Geometry check sheet. Reference: the model listing, model coordinates, mm. Coordinates: 2 decimals unless noted, no trailing zeros. Write each loop counter-clockwise with the first axis right and the second up, starting at its lowest first coordinate (ties: lowest second). Pieces come first, ordered by that corner, then holes. Notation, with made-up numbers: M 55.25,25.25 L 103.25,25.25 A22 cw 103.25,49.25 Z; hole C -38,50 d8. An arc over 180 degrees is marked long. Put each result on its own line as item: value. Start each with the question number.
1) Gauge pin test, flat ends, axial feed: pin 1 (1.1 mm diameter, centred on x = 78, z = 1, fed in from +Y); pin 2 (1.1 mm diameter, centred on y = 3.5, z = 1, fed in from +X); pin 3 (1.5 mm diameter, centred on y = 8, z = 0.5, fed in from -X); pin 4 (0.7 mm diameter, centred on x = 141.5, z = 0.5, fed in from -Y). Record the tip position at first contact, or that the pin passes through.
2) Scan lines: line 1 along Y through (x, z) = (68, 0.15); line 2 along X through (y, z) = (4, 1). Record each from-to range of solid material in increasing order.
3) Cross-section at C-C on z = 0.85. Record the cut outline in (x, y), plus the area to 3 significant figures.
4) Cross-section at A-A on x = 188. Record the cut outline in (y, z).
5) Cross-section at B-B on y = -3.5. Record the cut outline in (x, z).
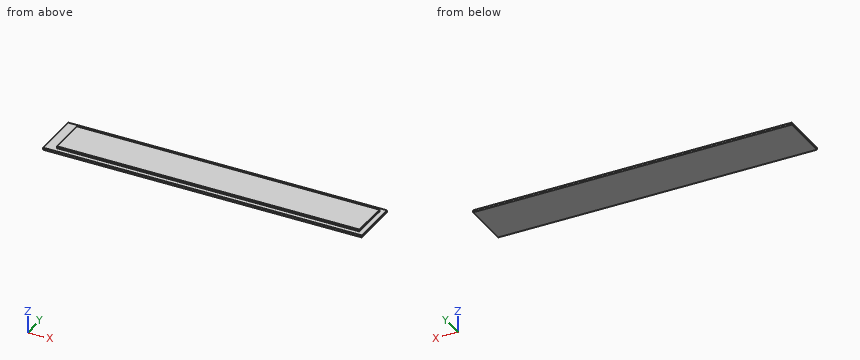
from build123d import *

# Parameters (mm, degrees)
SKETCH_1_W      = 226
SKETCH_1_H      = 34
SKETCH_1_W_2    = 214.5
SKETCH_1_H_2    = 27
EXTRUDE_1_DEPTH = 0.1
SKETCH_2_W      = 226
SKETCH_2_H      = 34
EXTRUDE_2_DEPTH = 1.4
SKETCH_3_W      = 214.5
SKETCH_3_H      = 27
EXTRUDE_3_DEPTH = 1.5


with BuildPart() as part:
    # Эскиз1 → Бобышка-Вытянуть1 (new body)
    with BuildSketch(Plane.XY):
        with Locations((108, 4.1)):
            Rectangle(SKETCH_1_W, SKETCH_1_H)
        with Locations((110.25, 4.1)):
            Rectangle(SKETCH_1_W_2, SKETCH_1_H_2, mode=Mode.SUBTRACT)
    extrude(amount=EXTRUDE_1_DEPTH)

    # Эскиз2 → Бобышка-Вытянуть2 (add)
    with BuildSketch(Plane(origin=(0, 0, 0), x_dir=(-1, 0, 0), z_dir=(0, 0, -1))):
        with Locations((-108, 4.1)):
            Rectangle(SKETCH_2_W, SKETCH_2_H)
    extrude(amount=EXTRUDE_2_DEPTH)

    # Эскиз3 → Бобышка-Вытянуть3 (add)
    with BuildSketch(Plane.XY):
        with Locations((110.25, 4.1)):
            Rectangle(SKETCH_3_W, SKETCH_3_H)
    extrude(amount=EXTRUDE_3_DEPTH)


solid = part.part
Answer key:
1. pin 1: stops at y = 17.6
1. pin 2: stops at x = 217.5
1. pin 3: stops at x = -5
1. pin 4: stops at y = -9.4
2. line 1: y = -9.4 to 17.6
2. line 2: x = 3 to 217.5
3. outline: M 3,-9.4 L 217.5,-9.4 L 217.5,17.6 L 3,17.6 Z
3. area: 5,790 mm²
4. outline: M -12.9,-1.4 L 21.1,-1.4 L 21.1,0.1 L 17.6,0.1 L 17.6,1.5 L -9.4,1.5 L -9.4,0.1 L -12.9,0.1 Z
5. outline: M -5,-1.4 L 221,-1.4 L 221,0.1 L 217.5,0.1 L 217.5,1.5 L 3,1.5 L 3,0.1 L -5,0.1 Z
